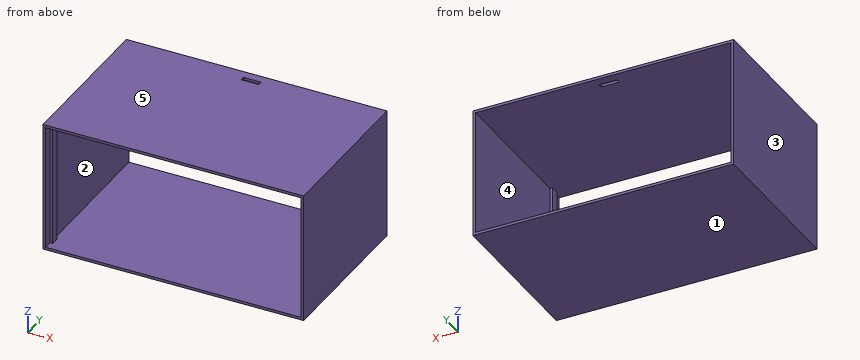
Autodesk Inventor part; units mm, degrees
ref_plane "YZ Plane" through (0, 0, 0) normal (1, 0, 0) x (0, 1, 0)
ref_plane "XZ Plane" through (0, 0, 0) normal (0, 1, 0) x (-1, 0, 0)
ref_plane "XY Plane" through (0, 0, 0) normal (0, 0, 1) x (1, 0, 0)
sketch "Szkic1" plane through (0, 0, 0) normal (0, 1, 0) x (-1, 0, 0)
  point P0 (0, 0)
sketch "Szkic2" plane through (0, 0, 0) normal (0, 1, 0) x (-1, 0, 0)
  line L0 (58.8, -28.8) -> (-58.8, -28.8)
  line L1 (-58.8, -28.8) -> (-58.8, 28.8)
  line L2 (-58.8, 28.8) -> (58.8, 28.8)
  line L3 (58.8, 28.8) -> (58.8, -28.8)
  line L4 (58.8, -28.8) -> (-58.8, 28.8) construction
  line L5 (-58.8, -28.8) -> (58.8, 28.8) construction
  line L6 (60, -30) -> (-60, -30)
  line L7 (-60, -30) -> (-60, 30)
  line L8 (-60, 30) -> (60, 30)
  line L9 (60, 30) -> (60, -30)
  line L10 (60, -30) -> (-60, 30) construction
  line L11 (-60, -30) -> (60, 30) construction
  line L12 (58.8, 28.8) -> (58.8, 30)
  point P0 (0, 0)
  dimension "d0" = 117.6
  dimension "d1" = 57.6
  dimension "d2" = 120
  dimension "d3" = 60
extrude "Wyciągnięcie proste1" add sketch "Szkic2" along normal blind 4
sketch "Szkic4" plane through (0, 4, 0) normal (0, 1, 0) x (1, 0, 0)
  line L0 (-60, 30) -> (60, 30)
  line L1 (60, 30) -> (60, -30)
  line L2 (60, -30) -> (-60, -30)
  line L3 (-60, -30) -> (-60, 30)
  line L4 (-60, 30) -> (60, -30) construction
  line L5 (60, 30) -> (-60, -30) construction
  line L6 (-57.6, 27.6) -> (57.6, 27.6)
  line L7 (57.6, 27.6) -> (57.6, -27.6)
  line L8 (57.6, -27.6) -> (-57.6, -27.6)
  line L9 (-57.6, -27.6) -> (-57.6, 27.6)
  line L10 (-57.6, 27.6) -> (57.6, -27.6) construction
  line L11 (57.6, 27.6) -> (-57.6, -27.6) construction
  line L12 (-57.6, 27.6) -> (-57.6, 30)
  point P0 (0, 0)
  dimension "d10" = 120
  dimension "d11" = 60
  dimension "d12" = 115.2
  dimension "d13" = 55.2
extrude "Wyciągnięcie proste2" add sketch "Szkic4" along normal blind 4
sketch "Szkic5" plane through (0, 8, 0) normal (0, 1, 0) x (1, 0, 0)
  line L0 (-58.8, 28.8) -> (58.8, 28.8)
  line L1 (58.8, 28.8) -> (58.8, -28.8)
  line L2 (58.8, -28.8) -> (-58.8, -28.8)
  line L3 (-58.8, -28.8) -> (-58.8, 28.8)
  line L4 (-58.8, 28.8) -> (58.8, -28.8) construction
  line L5 (58.8, 28.8) -> (-58.8, -28.8) construction
  line L6 (-60, 30) -> (60, 30)
  line L7 (60, 30) -> (60, -30)
  line L8 (60, -30) -> (-60, -30)
  line L9 (-60, -30) -> (-60, 30)
  line L10 (-60, 30) -> (60, -30) construction
  line L11 (60, 30) -> (-60, -30) construction
  line L12 (-58.8, 28.8) -> (58.8, 28.8)
  line L13 (-58.8, 28.8) -> (-58.8, 30)
  line L14 (60, 30) -> (-60, 30)
  point P0 (0, 0)
  dimension "d16" = 117.6
  dimension "d17" = 57.6
  dimension "d18" = 120
  dimension "d19" = 60
extrude "Wyciągnięcie proste3" add sketch "Szkic5" along normal blind 66
sketch "Szkic8" plane through (0, 4, 0) normal (0, -1, 0) x (1, 0, 0)
  line L0 (57.6, -28.8) -> (-57.6, -28.8)
  line L1 (-57.6, -28.8) -> (-57.6, 28.8)
  line L2 (-57.6, 28.8) -> (57.6, 28.8)
  line L3 (57.6, 28.8) -> (57.6, -28.8)
  line L4 (57.6, -28.8) -> (-57.6, 28.8) construction
  line L5 (-57.6, -28.8) -> (57.6, 28.8) construction
  point P0 (0, 0)
  dimension "d30" = 115.2
  dimension "d31" = 57.6
extrude "Wyciągnięcie proste5" cut sketch "Szkic8" against normal through all
sketch "Szkic9" plane through (-60, 0, 30) normal (0, 0, 1) x (1, 0, 0)
  line L0 (60, 0) -> (60, 69)
  line L1 (60, 0) -> (129, 0) construction
  line L2 (64, 68) -> (56, 68)
  line L3 (56, 68) -> (56, 70)
  line L4 (56, 70) -> (64, 70)
  line L5 (64, 70) -> (64, 68)
  line L6 (64, 68) -> (56, 70) construction
  line L7 (56, 68) -> (64, 70) construction
  dimension "d34" = 69
  dimension "d35" = 90
  dimension "d36" = 8
  dimension "d37" = 2
extrude "Wyciągnięcie proste6" cut sketch "Szkic9" against normal blind 10
properties part number "sciany boczne"
Can you work these out from the model? Positions are in its coordinate system, mm. Face numbers are marked on the shaded views. A direction names the side the tool comes from. Coordinates: 2 decimals unless noted, no trailing zeros. Loops run counter-clockwise (first coordinate to the right, second up) from the corner with the lowest first, then second, coordinate; pieces in that order, holes last.
1) I need wall thicknesses on probe 1 along X at (y, z) = (62, -15); probe 2 along X at (y, z) = (7, 10.5); probe 3 along Z at (x, y) = (-13, 8.5). Which ranges of each line are inside material? Lowest first, please.
2) Imagine slicing it at C-C on y = 44. List the corners of the cut face in (x, z) for me.
3) Which directions (+Z, -Z, +X, -X, +Y, -Y) give clear straight access to the entire face, cutting with the end or side of a thin tool? Please do the marked faces 4 and 5.
4) Imagine slicing it at B-B on z = -11. List the corners of the cut face in (x, y) for me, plus the area to 3 significant figures.
5) For pin 1 (0.6 mm diameter, centred on x = 58, z = -12.5, fed in from -Y); pin 2 (1 mm diameter, centred on x = 58, z = -6, fed in from +Y), each with a flat end and sliding along its axis, tell me the tip position at first contact or that it passes through.
6) Thinking about a two-plate mould opening in Z: for the marked faces 1, 2 and 3, which applies, pulls with the +Z half, pulls with the -Z half, needs draft (parallel to the pull), parting line crosses it, or undercut?
7) Imagine slicing it at A-A on x = 36. List the corners of the cut face in (y, z) for me.
Completed:
1. probe 1: x = -60 to -58.8, 58.8 to 60
1. probe 2: x = -60 to -57.6, 57.6 to 60
1. probe 3: z = -30 to -28.8, 28.8 to 30
2. outline: (-60, -30) - (60, -30) - (60, 30) - (-60, 30) - close; hole (-58.8, -28.8) - (58.8, -28.8) - (58.8, 28.8) - (-58.8, 28.8) - close
3. face 4: +Y
3. face 5: +Z, +X, -X, +Y, -Y
4. outline: (-60, 0) - (-58.8, 0) - (-58.8, 4) - (-57.6, 4) - (-57.6, 8) - (-58.8, 8) - (-58.8, 74) - (-60, 74) - close; (57.6, 4) - (58.8, 4) - (58.8, 0) - (60, 0) - (60, 74) - (58.8, 74) - (58.8, 8) - (57.6, 8) - close
4. area: 187 mm2
5. pin 1: stops at y = 4
5. pin 2: stops at y = 8
6. face 1: pulls with the -Z half
6. face 2: undercut
6. face 3: needs draft
7. outline: (0, -30) - (74, -30) - (74, -28.8) - (0, -28.8) - close; (0, 28.8) - (74, 28.8) - (74, 30) - (0, 30) - close
